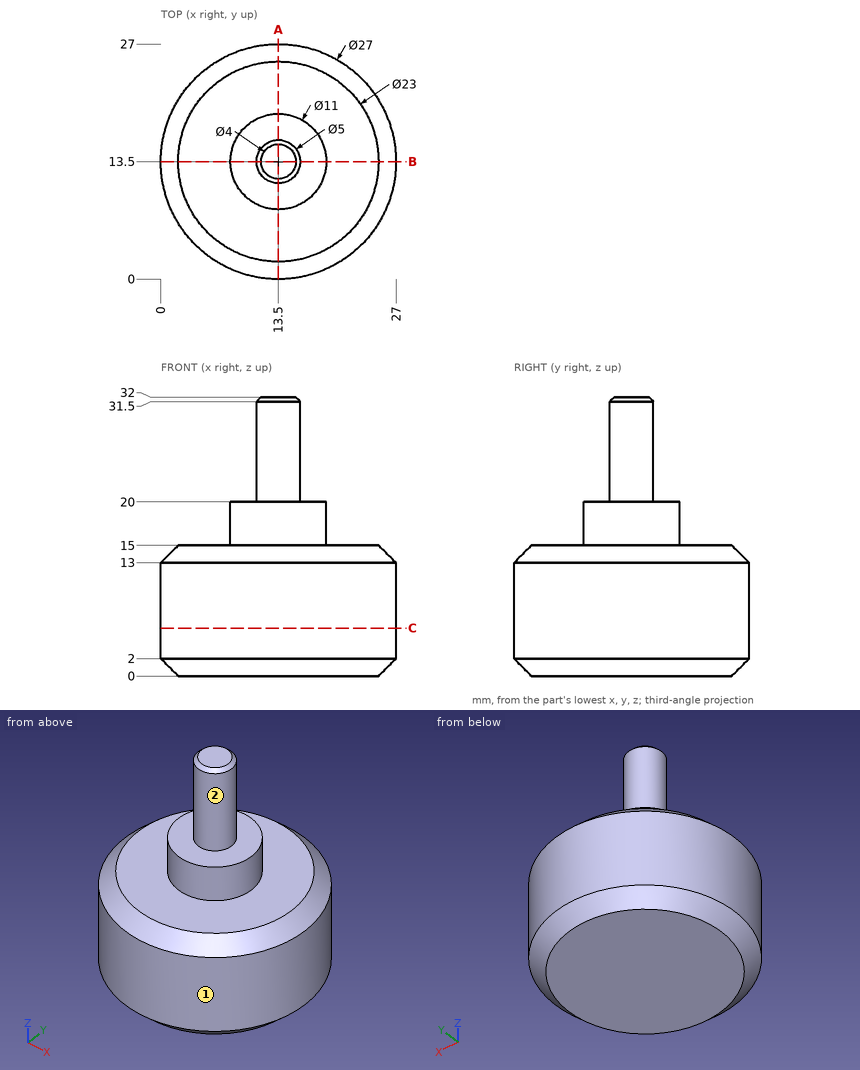
Study the drawing (mm; zero at the part's minimum x, y, z) and answer. A direction names the side the tool comes from. Give positions to 0.01 mm unless a question says otherwise; leave off trailing zeros. Order: outer loops, then holes, each group sorted by start corner. A loop starts at its lowest first (then second) coordinate and runs counter-clockwise, first axis right, second up. Notation, with made-up numbers: M -6,7 L 29,7 A31 cw 29,31 Z; hole C 9,80.5 d4. An arc over 180 degrees is marked long. Put each result on its own line as item: value. Start each with the question number.
Item 1: Which of the six approach directions +Z, -Z, +X, -X, +Y, -Y give full straight-line access (tool end or side, diameter ignored) to the marked faces 1 and 2?
Item 2: The part is cut by section C-C, the plane z = 5.5. Determine the outline of the cut face in (x, y), and give its area (3 significant figures).
Item 3: Flat-ended cylindrical pins translate along their axes: P1, Ø8, axis at x = 7.5, z = 15.5, coming from the +Y side; P2, Ø5, axis at x = 5.5, y = 5.5, coming from the -Z side; P3, Ø3, axis at x = 11, y = 8, coming from the +Z side; P4, Ø8, axis at x = 21, z = 5.5, coming from the +Y side. Find the tip coordinate at first contact, or state that the pin passes through.
Item 4: The part is cut by section A-A, the plane x = 13.5. Determine the outline of the cut face in (y, z).
Item 5: Find the intervals of material crossed by line 1 along Z through (x, y) = (12.25, 2.75); line 2 along X through (y, z) = (15, 23.5); line 3 along Y through (x, z) = (14, 14.5), in increasing order.
Answer key:
1. face 1: +Z, -Z
1. face 2: +Z
2. outline: C 13.5,13.5 d27
2. area: 573 mm²
3. P1: stops at y = 26.69
3. P2: stops at z = 0
3. P3: stops at z = 20
3. P4: stops at y = 26.54
4. outline: M 0,2 L 2,0 L 25,0 L 27,2 L 27,13 L 25,15 L 19,15 L 19,20 L 16,20 L 16,31.5 L 15.5,32 L 11.5,32 L 11,31.5 L 11,20 L 8,20 L 8,15 L 2,15 L 0,13 Z
5. line 1: z = 0 to 15
5. line 2: x = 11.5 to 15.5
5. line 3: y = 1.51 to 25.49
